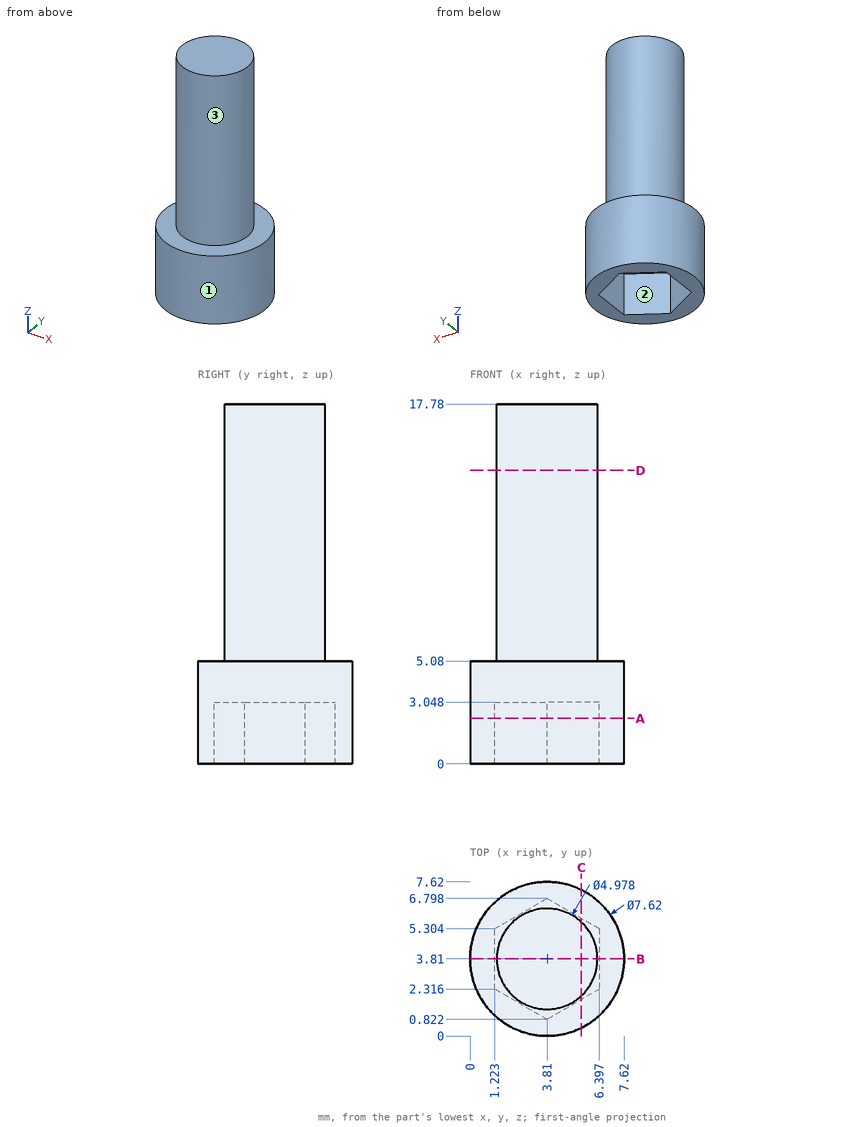
Study the drawing (mm; zero at the part's minimum x, y, z) and answer. A direction names the side the tool comes from. Coordinates: 2 decimals unless noted, no trailing zeros. Write each loop counter-clockwise with the first axis right and the second up, starting at its lowest first coordinate (ties: lowest second). Pieces come first, ordered by that corner, then holes. Notation, with made-up numbers: M 5,-19 L 34,-19 A27 ccw 34,11 Z; hole C 57.25,35 d9. An arc over 180 degrees is marked long. Use a Markdown table: item, result. Add a question column.
1. Section D-D (z = 14.5) is taken. Give the vertices of the cut face in (x, y), plus the area to 3 significant figures.
2. Which of the six approach directions +Z, -Z, +X, -X, +Y, -Y give full straight-line access (tool end or side, diameter ignored) to the marked faces 1, 2 and 3?
3. Given P1, Ø2.5, axis at x = 4, y = 4.5, coming from the -Z side; P2, Ø1, axis at y = 4, z = 14, coming from the +X side; P3, Ø4, axis at y = 4, z = 14.5, coming from the -X side, each flat-ended and moving along its own axis, determine where each tip first touches the part or whether it passes through.
4. Section B-B (y = 3.81) is taken. Give the vertices of the cut face in (x, z).
5. Straight lines are drawn through the part: line 1 along Z through (x, y) = (3, 5.5); line 2 along X through (y, z) = (4.5, 1.5); line 3 along Y through (x, z) = (3.75, 15.75). For each, find the intervals that lie inside material, in ascending order. Write a range as [from, to].
6. Section C-C (x = 5.5) is taken. Give the vertices of the cut face in (y, z) (1 decimal).
7. Section A-A (z = 2.25) is taken. Give the vertices of the cut face in (x, y).
Data:
| question | item | result |
|---|---|---|
| 1 | outline | C 3.81,3.81 d4.98 |
| 1 | area | 19.5 mm2 |
| 2 | face 1 | +Z, -Z |
| 2 | face 2 | -Z |
| 2 | face 3 | +Z |
| 3 | P1 | stops at z = 3.05 |
| 3 | P2 | stops at x = 6.3 |
| 3 | P3 | stops at x = 1.32 |
| 4 | outline | M 0,0 L 1.22,0 L 1.22,3.05 L 6.4,3.05 L 6.4,0 L 7.62,0 L 7.62,5.08 L 6.3,5.08 L 6.3,17.78 L 1.32,17.78 L 1.32,5.08 L 0,5.08 Z |
| 5 | line 1 | z = [3.05, 17.78] |
| 5 | line 2 | x = [0.06, 1.22], [6.4, 7.56] |
| 5 | line 3 | y = [1.32, 6.3] |
| 6 | outline | M 0.4,0 L 1.8,0 L 1.8,3 L 5.8,3 L 5.8,0 L 7.2,0 L 7.2,5.1 L 5.6,5.1 L 5.6,17.8 L 2,17.8 L 2,5.1 L 0.4,5.1 Z |
| 7 | outline | C 3.81,3.81 d7.62; hole M 1.22,2.32 L 3.81,0.82 L 6.4,2.32 L 6.4,5.3 L 3.81,6.8 L 1.22,5.3 Z |
